Verification items for the finished model (mm, model axes). Face numbers are marked on the shaded views. Give positions to 0.01 mm unless a question says otherwise; leave off trailing zeros. Loops run counter-clockwise (first coordinate to the right, second up) from the corner with the lowest first, then second, coordinate; pieces in that order, holes last. Notation, with made-up numbers: M -11,-21 L -5,-21 A33 cw -5,18 Z; hole C 39,37 d9. An arc over 180 degrees is marked long. Answer in a Markdown table with one row per item.
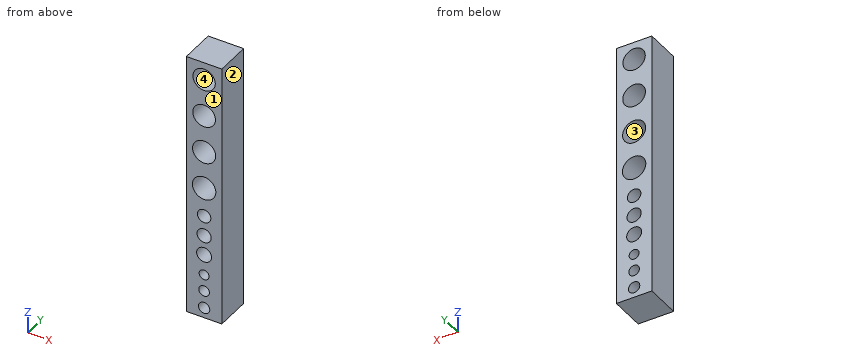
Autodesk Inventor part; units mm, degrees
ref_plane "YZ Plane" through (0, 0, 0) normal (1, 0, 0) x (0, 1, 0)
ref_plane "XZ Plane" through (0, 0, 0) normal (0, 1, 0) x (-1, 0, 0)
ref_plane "XY Plane" through (0, 0, 0) normal (0, 0, 1) x (1, 0, 0)
sketch "Szkic1" plane through (0, 0, 0) normal (0, 1, 0) x (-1, 0, 0)
  line L0 (0, 0) -> (10, 0)
  line L1 (10, 0) -> (10, -75)
  line L2 (10, -75) -> (0, -75)
  line L3 (0, -75) -> (0, 0)
  circle A0 centre (5, -5) radius 3.15
  circle A1 centre (5, -15.6324) radius 3.2
  circle A2 centre (5, -26.2648) radius 3.25
  circle A3 centre (5, -36.8972) radius 3.3
  line L4 (5, -5) -> (5, -15.6324) construction
  line L5 (5, -15.6324) -> (5, -26.2648) construction
  line L6 (5, -26.2648) -> (5, -36.8972) construction
  circle A4 centre (5, -45.1205) radius 1.9
  circle A5 centre (5, -56.4925) radius 2.1
  circle A6 centre (5, -50.8625) radius 2
  circle A7 centre (5, -62.3904) radius 1.4
  circle A8 centre (5, -67.132) radius 1.5
  circle A9 centre (5, -72.0899) radius 1.6
  line L7 (5, -36.8972) -> (5, -75) construction
  dimension "d0" = 10
  dimension "d1" = 75
  dimension "d2" = 6.3
  dimension "d3" = 6.4
  dimension "d4" = 6.5
  dimension "d5" = 6.6
  dimension "d6" = 5
  dimension "d7" = 3.8
  dimension "d8" = 4.2
  dimension "d9" = 4
  dimension "d12" = 2.8
  dimension "d13" = 3
  dimension "d14" = 3.2
extrude "Wyciągnięcie proste1" add sketch "Szkic1" along normal blind 10
properties part number "test_print"
Item 1: Sectioned sample at B-B (x = -5). State how many separate pieces and enclosed holes the cut face has, and give its area (3 significant figures).
Reported:
| item | result |
|---|---|
| separate pieces | 11 |
| enclosed holes | 0 |
| area | 282 mm^2 |
Item 2: Scan lines: L1, parallel to X at y = 4.5, z = -37.5; L2, parallel to X at y = 9.5, z = -14.5; L3, parallel to Z at x = -2.75, y = 2.5. Record each from-to range of solid material in increasing order. Write a range as [from, to].
Reported:
| item | result |
|---|---|
| L1 | x = [-10, -8.24], [-1.76, 0] |
| L2 | x = [-10, -7.99], [-2.01, 0] |
| L3 | z = [-75, -39.31], [-34.48, -28.61], [-23.92, -17.91], [-13.36, -7.2], [-2.8, 0] |
Item 3: Sectioned sample at A-A (z = -5). Record the cut outline in (x, y).
Reported:
| item | result |
|---|---|
| outline | M -10,0 L -8.15,0 L -8.15,10 L -10,10 Z; M -1.85,0 L 0,0 L 0,10 L -1.85,10 Z |
Item 4: Sectioned sample at D-D (z = -39). Record the cut outline in (x, y), and give its area (3 significant figures).
Reported:
| item | result |
|---|---|
| outline | M -10,0 L -7.54,0 L -7.54,10 L -10,10 Z; M -2.46,0 L 0,0 L 0,10 L -2.46,10 Z |
| area | 49.1 mm^2 |
Item 5: Release check for a two-part mould opening along X. For the marked faces 1, 2, 3 and 4 record: released by +X, released by -X, zero draft, split by the parting line, or undercut.
Reported:
| item | result |
|---|---|
| face 1 | zero draft |
| face 2 | released by +X |
| face 3 | undercut |
| face 4 | undercut |
Item 6: Go/stop test with flat-tipped pins: pin 1 (2 mm diameter, centred on x = -5.5, z = -56.5, fed in from +Y); pin 2 (3 mm diameter, centred on y = 3.5, z = -16, fed in from +X). Record where each tip stops, or that it passes through.
Reported:
| item | result |
|---|---|
| pin 1 | passes through |
| pin 2 | stops at x = 0 |
